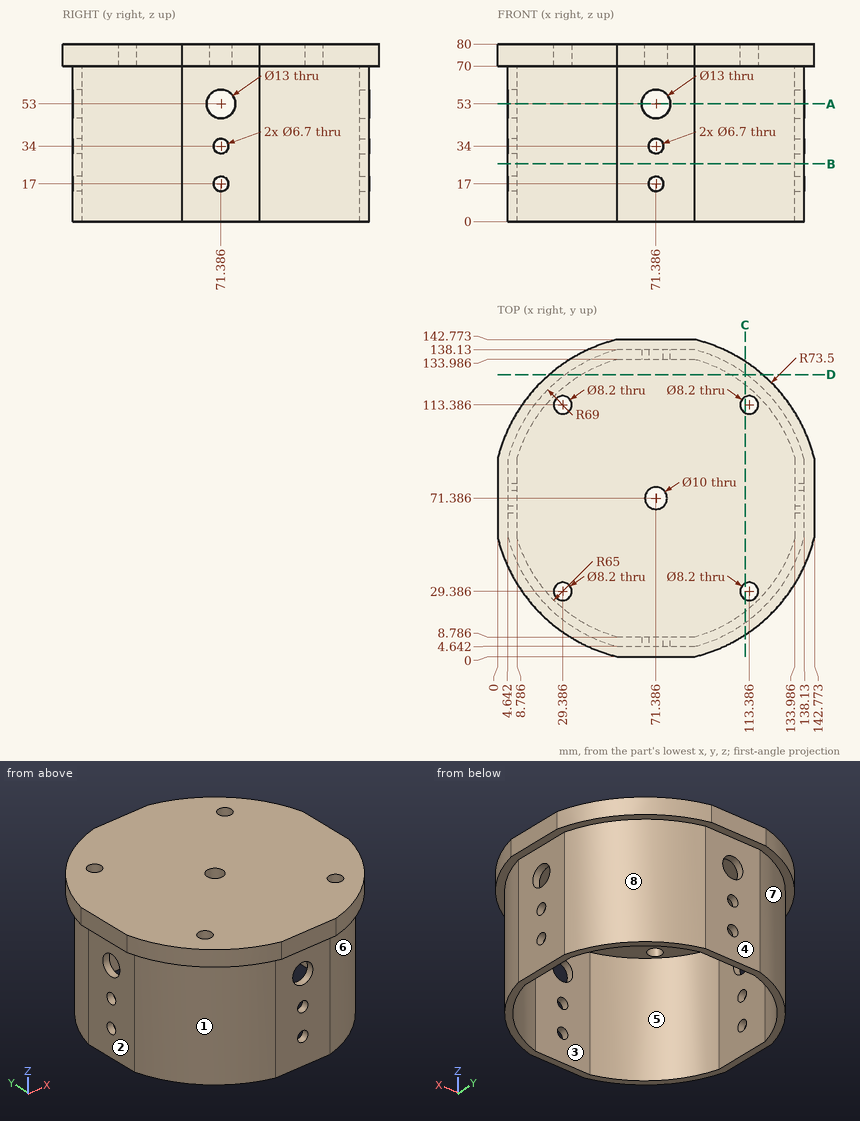
Here's the drawing with two shaded views (mm, measured from the low corner). I have some questions. A direction names the side the tool comes from. Coordinates: 2 decimals unless noted, no trailing zeros. Loops run counter-clockwise (first coordinate to the right, second up) from the corner with the lowest first, then second, coordinate; pieces in that order, holes last. Notation, with made-up numbers: (3.25, -38.5) -> (33.25, -38.5) arc R25 ccw to (33.25, -18.5) -> close; hole circle Ø6 at (64, -29). An arc over 180 degrees is marked (long way). Answer as a JSON object with one key per item and string values.
1) Thinking about a two-plate mould opening in Y: for the marked faces 1, 2 and 3, which applies, pulls with the +Y half, pulls with the -Y half, needs draft (parallel to the pull), parting line crosses it, or undercut?
Results:
{"face 1": "pulls with the -Y half", "face 2": "needs draft", "face 3": "undercut"}
2) If I drill on line 1 (Y direction, x = 60, z = 5); line 2 (X direction, y = 114, z = 46) (1 decimal), over which ranges is the centre line in solid material (lowest first)?
Results:
{"line 1": "y = 4.64 to 8.79, 133.99 to 138.13", "line 2": "x = 17.1 to 22.3, 120.5 to 125.7"}
3) For P1, Ø6.5, axis at x = 29.39, y = 29.39, coming from the +Z side; P2, Ø1.5, axis at x = 96, y = 15.5, coming from the -Z side; P3, Ø6, axis at x = 96.5, z = 37, coming from the -Y side (1 decimal); P4, Ø8, axis at x = 31.5, z = 15.5, coming from the +Y side, each with a flat end and sliding along its axis, tell me the tip position at first contact or that it passes through.
Results:
{"P1": "passes through", "P2": "stops at z = 70", "P3": "stops at y = 6", "P4": "stops at y = 130.32"}
4) Imagine slicing it at C-C (x = 111.5). Please give me the cut outline in (y, z) (1 decimal).
Results:
{"outline": "(9.8, 70) -> (15.2, 70) -> (15.2, 0) -> (20.2, 0) -> (20.2, 70) -> (25.7, 70) -> (25.7, 80) -> (9.8, 80) -> close; (33, 70) -> (109.7, 70) -> (109.7, 80) -> (33, 80) -> close; (117, 70) -> (122.5, 70) -> (122.5, 0) -> (127.5, 0) -> (127.5, 70) -> (133, 70) -> (133, 80) -> (117, 80) -> close"}
5) Imagine slicing it at A-A (z = 53). Count the separate pieces of the cut face and the enclosed holes in it, then the cut area to 3 significant figures.
Results:
{"separate pieces": "4", "enclosed holes": "0", "area": "1,480 mm^2"}
6) Imagine slicing it at D-D (y = 127). Please give me the cut outline in (x, z).
Results:
{"outline": "(23.33, 70) -> (30.54, 70) -> (30.54, 0) -> (37.74, 0) -> (37.74, 70) -> (105.03, 70) -> (105.03, 0) -> (112.23, 0) -> (112.23, 70) -> (119.44, 70) -> (119.44, 80) -> (23.33, 80) -> close"}
7) For the marked faces 4, 5, 6, 7 and 8, which set-ups out of +Z, -Z, +X, -X, +Y, -Y let a thin tool reach every point of the face, with its end or its side?
Results:
{"face 4": "-Z, +X, -X, +Y", "face 5": "-Z", "face 6": "-Z, +X, -Y", "face 7": "-Z, -X, +Y", "face 8": "-Z, +X, +Y"}
8) Imagine slicing it at B-B (z = 26). Please give me the cut outline in (x, y), then the cut area to 3 significant figures.
Results:
{"outline": "(4.64, 53.89) arc R69 ccw to (53.89, 4.64) -> (88.89, 4.64) arc R69 ccw to (138.13, 53.89) -> (138.13, 88.89) arc R69 ccw to (88.89, 138.13) -> (53.89, 138.13) arc R69 ccw to (4.64, 88.89) -> close; hole (8.79, 53.89) arc R65 ccw to (53.89, 8.79) -> (88.89, 8.79) arc R65 ccw to (133.99, 53.89) -> (133.99, 88.89) arc R65 ccw to (88.89, 133.99) -> (53.89, 133.99) arc R65 ccw to (8.79, 88.89) -> close", "area": "1,700 mm^2"}
